Geometry: final body of the model. Coordinates: model frame, mm. Face numbers are marked on the shaded views. A direction names the side the tool comes from. Give positions to 0.01 mm unless a question says otherwise; leave off trailing zeros. Order: outer loops, then holes, each group sorted by start corner. A loop starts at its lowest first (then second) coordinate and runs counter-clockwise, first axis right, second up. Notation, with made-up numbers: (-16.75, -3.5) - (21.25, -3.5) arc R30 ccw to (21.25, 18.5) - close; hole circle Ø10 at (87.25, -10.75). An arc over 180 degrees is marked (long way). Use one line per item in the form item = value.
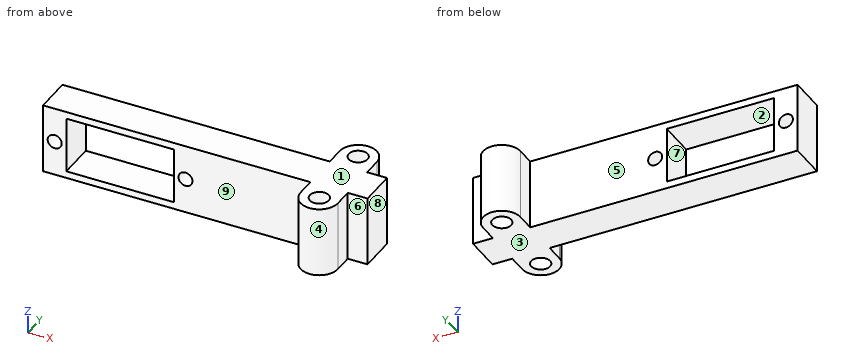
Autodesk Inventor part; units mm, degrees
ref_plane "YZ Plane" through (0, 0, 0) normal (1, 0, 0) x (0, 1, 0)
ref_plane "XZ Plane" through (0, 0, 0) normal (0, 1, 0) x (-1, 0, 0)
ref_plane "XY Plane" through (0, 0, 0) normal (0, 0, 1) x (1, 0, 0)
sketch "Sketch1" plane through (0, 0, 0) normal (0, 1, 0) x (-1, 0, 0)
  line L0 (-25.5949, 6.1189) -> (0.4051, 6.1189)
  line L1 (-25.5949, 6.1189) -> (0.4051, 6.1189)
  line L2 (0.4051, 6.1189) -> (0.4051, -8.8811)
  line L3 (0.4051, -8.8811) -> (-25.5949, -8.8811)
  line L4 (-25.5949, -8.8811) -> (-25.5949, 6.1189)
  line L5 (0.4051, -8.8811) -> (27.4051, -8.8811)
  line L6 (27.4051, -8.8811) -> (27.4051, 6.1189)
  line L7 (27.4051, 6.1189) -> (0.4051, 6.1189)
  line L8 (0.4051, 6.1189) -> (0.4051, -8.8811)
  line L9 (22.4051, -1.3811) -> (22.4051, -7.3811)
  line L10 (22.4051, -7.3811) -> (22.4051, 4.6189)
  line L11 (22.4051, 4.6189) -> (-0.5949, 4.6189)
  line L12 (-0.5949, 4.6189) -> (-0.5949, -7.3811)
  line L13 (-0.5949, -7.3811) -> (22.4051, -7.3811)
  line L14 (22.4051, -1.3811) -> (27.4051, -1.3811)
  circle A0 centre (24.9051, -1.3811) radius 1.5
  line L15 (-0.5949, -1.3811) -> (-5.5949, -1.3811)
  circle A1 centre (-3.0949, -1.3811) radius 1.5
  point P0 (0, 0)
  dimension "d0" = 15
  dimension "d1" = 27
  dimension "d2" = 5
  dimension "d3" = 6
  dimension "d4" = 12
  dimension "d5" = 23
  dimension "d6" = 5
  dimension "d7" = 3
  dimension "d8" = 5
  dimension "d9" = 3
extrude "Extrusion1" add sketch "Sketch1" along normal blind 8 contours L0 L2 L11 L12 L13 L3 L4 | L7 L6 L14 A0 L10 L11 L2 | L2 L13 L9 L14 A0 L6 L5
sketch "Sketch4" plane through (-27.4051, 0, 6.1189) normal (0, 0, 1) x (1, 0, 0)
  line L0 (53, 8) -> (69.5, 8)
  line L1 (69.5, 8) -> (69.5, 0)
  line L2 (69.5, 0) -> (53, 0)
  line L3 (53, 0) -> (53, 8)
  point P0 (27.4051, 0)
  dimension "d24" = 16.5
extrude "Extrusion3" add sketch "Sketch4" against normal up to surface (15 mm away)
sketch "Sketch5" plane through (-27.4051, 0, 6.1189) normal (0, 0, 1) x (1, 0, 0)
  line L0 (69.5, 0) -> (69.5, 8)
  line L1 (69.5, 0) -> (69.5, 8)
  line L2 (61.25, 4) -> (61.25, 12)
  line L3 (61.25, 12) -> (61.25, -4)
  circle A0 centre (61.25, 12) radius 2.025
  circle A1 centre (61.25, -4) radius 2.025
  circle A2 centre (61.25, 12) radius 4
  circle A3 centre (61.25, -4) radius 4
  line L4 (57.25, 12) -> (57.25, -4)
  line L5 (65.25, -4) -> (65.25, 12)
  point P0 (27.4051, 0)
  point P1 (69.5, 4)
  point P2 (69.5, 4)
  dimension "d27" = 8.25
  dimension "d28" = 8
  dimension "d29" = 16
  dimension "d30" = 4.05
  dimension "d31" = 4.05
  dimension "d32" = 8
  dimension "d33" = 8
extrude "Extrusion4" add sketch "Sketch5" against normal up to surface (15 mm away)
properties part number "servo_holder_3DPrint"
(1) Cut plane C-C on y = 5.75. Output: boundary loops of the cut face in (x, z).
Computed values:
outline = (-27.41, -8.88) - (42.09, -8.88) - (42.09, 6.12) - (-27.41, 6.12) - close; hole circle Ø3 at (-24.91, -1.38); hole (-22.41, -7.38) - (0.59, -7.38) - (0.59, 4.62) - (-22.41, 4.62) - close; hole circle Ø3 at (3.09, -1.38)
(2) Cut plane B-B on x = -0.5. Output: boundary loops of the cut face in (y, z), plus the area to 3 significant figures.
Computed values:
outline = (0, -8.88) - (8, -8.88) - (8, -7.38) - (0, -7.38) - close; (0, 4.62) - (8, 4.62) - (8, 6.12) - (0, 6.12) - close
area = 24.0 mm²
(3) Ray query, line 1 along Z through (x, y) = (-19, 6.25); line 2 along Y through (x, z) = (32, -3.5); line 3 along X through (y, z) = (-4, 0.25). Return the intervals inside material, ascending.
Computed values:
line_1 = -8.88 to -7.38, 4.62 to 6.12
line_2 = -7.55 to -4.83, -3.17 to 11.17, 12.83 to 15.55
line_3 = 29.84 to 31.82, 35.87 to 37.84
(4) Cut plane D-D on x = 29. Output: boundary loops of the cut face in (y, z), plus the area to 3 significant figures.
Computed values:
outline = (0, -8.88) - (8, -8.88) - (8, 6.12) - (0, 6.12) - close
area = 120 mm²
(5) Contact query for flat-ended pins moving along their axis: pin 1 Ø1.8 at (x, z) = (3.09, -1.38) entering from +Y; pin 2 Ø1.5 at (y, z) = (-1.5, -6.5) entering from +X; pin 3 Ø6 at (x, y) = (-15, 8.5) entering from +Z; pin 4 Ø1 at (x, z) = (24, 0) entering from -Y. Output: stop coordinate, or through.
Computed values:
pin_1 = through
pin_2 = 37.84
pin_3 = 6.12
pin_4 = 0
(6) Pull-direction query (Z, two-part tool) for the marked faces 1, 2, 3 and 4; classes: released by +Z, released by -Z, zero draft, split by the parting line, or undercut.
Computed values:
face_1 = released by +Z
face_2 = undercut
face_3 = released by -Z
face_4 = zero draft
(7) Cut plane A-A on z = -4. Output: boundary loops of the cut face in (x, y) (3 decimals), plus the area to 4 significant figures.
Computed values:
outline = (-27.405, 0) - (-22.405, 0) - (-22.405, 8) - (-27.405, 8) - close; (0.595, 0) - (29.845, 0) - (29.845, -4) arc R4 ccw to (37.845, -4) - (37.845, 0) - (42.095, 0) - (42.095, 8) - (37.845, 8) - (37.845, 12) arc R4 ccw to (29.845, 12) - (29.845, 8) - (0.595, 8) - close; hole circle Ø4.05 at (33.845, -4); hole circle Ø4.05 at (33.845, 12)
area = 460.5 mm²
(8) Reachability of the marked faces 5, 6, 7, 8 and 9 from +Z, -Z, +X, -X, +Y, -Y: full face, straight path, thin tool, end or side. Return the list, or none.
Computed values:
face_5 = +Z, -Z, -X, +Y
face_6 = +Z, -Z, +X, -Y
face_7 = +Y, -Y
face_8 = +Z, -Z, +X, +Y, -Y
face_9 = +Z, -Z, -X, -Y
